The listing builds one solid part. Answer for the finished solid, in the listing's coordinates (mm). Face numbers are marked on the shaded views. Round coordinates to 2 decimals unless told otherwise and drop trailing zeros. Loops run counter-clockwise (first coordinate to the right, second up) from the corner with the lowest first, then second, coordinate; pieces in that order, holes last. Notation, with made-up numbers: (72.5, 1) -> (86.5, 1) arc R13 cw to (86.5, 14) -> close; hole circle Ø11 at (32, 44). An arc over 180 degrees is marked (long way). Answer in a Markdown table with one row per item. Add a question column.
```python
from build123d import *

# Parameters (mm, degrees)
F1_DEPTH = 50.8


with BuildPart() as f1:
    # F0 (on Front) → F1 (new body)
    with BuildSketch(Plane.XZ):
        with BuildLine():
            Line((-128.940001, -9.03), (-120.54, -14.07))
            Line((-120.54, -14.07), (-98.700002, -14.07))
            ThreePointArc((-98.700002, -14.07), (-91.116523, -3.930836), (-78.540005, -5.394729))
            Line((-78.540005, -5.394729), (-78.540005, 11.130001))
            Line((-78.540005, 11.130001), (-128.940001, -9.03))
        make_face()
        with BuildLine():
            Line((-78.540005, 11.130001), (-78.540005, -5.394729))
            ThreePointArc((-78.540005, -5.394729), (-75.12633, -9.213174), (-73.5, -14.07))
            Line((-73.5, -14.07), (-34.44, -14.07))
            Line((-34.44, -14.07), (-34.44, 11.130001))
            Line((-34.44, 11.130001), (-78.540005, 11.130001))
        make_face()
        Polygon((-59.220001, 22.89), (-78.540005, 11.130001), (-34.44, 11.130001), (-6.562005, 11.130001), (13.203657, 11.130001), (-9.659999, 22.89), align=None)
        with BuildLine():
            Line((-6.562005, 11.130001), (-34.44, 11.130001))
            Line((-34.44, 11.130001), (-34.44, -14.07))
            Line((-34.44, -14.07), (-25.1968, -14.07))
            ThreePointArc((-25.1968, -14.07), (-17.621716, -5.998406), (-6.562005, -6.462444))
            Line((-6.562005, -6.462444), (-6.562005, 11.130001))
        make_face()
        with BuildLine():
            Line((13.203657, 11.130001), (-6.562005, 11.130001))
            Line((-6.562005, 11.130001), (-6.562005, -6.462444))
            ThreePointArc((-6.562005, -6.462444), (-2.534474, -9.622293), (0, -14.07))
            Line((0, -14.07), (7.139999, -14.07))
            Line((7.139999, -14.07), (19.737999, 0))
            Line((19.737999, 0), (19.737999, 7.769039))
            Line((19.737999, 7.769039), (13.203657, 11.130001))
        make_face()
    extrude(amount=F1_DEPTH)


solid = f1.part
```
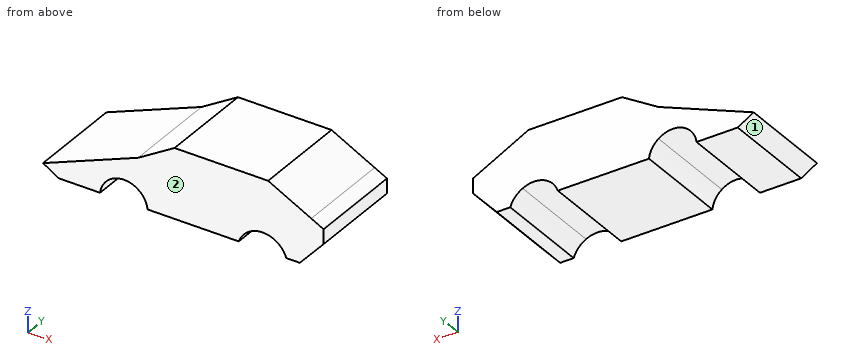
Item 1: The mould has two halves that part along X. Classify the marked faces 1 and 2: +X half, -X half, draft (parallel to the pull), parting line (faces both ways), or undercut.
Item 2: Section A-A, the plane y = -43.5 is taken. Write down the section's boundary in (x, z).
Item 3: Section C-C, the plane x = -11 is taken. Write down the section's boundary in (y, z), and give its area (3 significant figures).
Item 4: Section B-B, the plane z = 13.5 is taken. Write down the section's boundary in (x, y).
Item 5: Flat-ended cylindrical pins translate along their axes: P1, Ø5, axis at y = -8, z = 13, coming from the +X side; P2, Ø1.5, axis at y = -21, z = 9, coming from the -X side; P3, Ø4, axis at x = -6.5, y = -13, coming from the +Z side. Find the tip coordinate at first contact, or state that the pin passes through.
Item 6: Consider L1, parallel to X at y = -30, z = -9.5; L2, parallel to Z at x = -97, y = -24; L3, parallel to Z at x = -14, y = -26. Determine where each line is inside the solid, lowest interval first. Write a range as from..to.
Here are the results:
| question | item | result |
|---|---|---|
| 1 | face 1 | -X half |
| 1 | face 2 | draft |
| 2 | outline | (-128.94, -9.03) -> (-120.54, -14.07) -> (-98.7, -14.07) arc R12.69 cw to (-78.54, -5.39) arc R12.69 cw to (-73.5, -14.07) -> (-25.2, -14.07) arc R13.29 cw to (-6.56, -6.46) arc R13.29 cw to (0, -14.07) -> (7.14, -14.07) -> (19.74, 0) -> (19.74, 7.77) -> (13.2, 11.13) -> (-9.66, 22.89) -> (-59.22, 22.89) -> (-78.54, 11.13) -> close |
| 3 | outline | (-50.8, -5.11) -> (0, -5.11) -> (0, 22.89) -> (-50.8, 22.89) -> close |
| 3 | area | 1,420 mm² |
| 4 | outline | (-74.65, -50.8) -> (8.6, -50.8) -> (8.6, 0) -> (-74.65, 0) -> close |
| 5 | P1 | stops at x = 14.43 |
| 5 | P2 | stops at x = -85.74 |
| 5 | P3 | stops at z = 22.29 |
| 6 | L1 | x = -128.16..-97.24, -74.96..-22.56, -2.64..11.23 |
| 6 | L2 | z = -9.09..3.75 |
| 6 | L3 | z = -5.09..22.89 |
